Geometry check sheet. Reference: the model listing, model coordinates, mm. Give positions to 0.01 mm unless a question says otherwise; leave off trailing zeros. Order: outer loops, then holes, each group sorted by start corner. A loop starts at its lowest first (then second) coordinate and runs counter-clockwise, first axis right, second up.
```python
from build123d import *

# Parameters (mm, degrees)
F0_R           = 27.4134107223
F1_DEPTH       = 25
F2_R           = 5
F3_DEPTH       = 25
F3_DEPTH_BACK  = 25
F4_R           = 5
F5_R           = 5.7754961782
F6_DEPTH       = 27.4144107223
F6_DEPTH_BACK  = 27.4144107223
F9_R           = 5
F10_DEPTH      = 38.7694173758
F10_DEPTH_BACK = 38.7694173758


with BuildPart() as f1:
    # F0 (on Front) → F1 (new body)
    with BuildSketch(Plane.XZ):
        Circle(F0_R)
    extrude(amount=F1_DEPTH)

    # F2 (on face) → F3 (cut, two sides)
    with BuildSketch(Plane.XZ.offset(25)) as f3_sk:
        with Locations((0, -0.6682850071)):
            Circle(F2_R)
    extrude(amount=-F3_DEPTH, mode=Mode.SUBTRACT)
    extrude(f3_sk.sketch, amount=F3_DEPTH_BACK, mode=Mode.SUBTRACT)

    # F4
    f4_edges = [f1.edges().sort_by_distance(p)[0] for p in [
        (-5, -25, -0.668285),
    ]]
    fillet(f4_edges, radius=F4_R)

    # F5 (on Right) → F6 (cut, two sides)
    with BuildSketch(Plane.YZ) as f6_sk:
        with Locations((-12.5455856323, 0)):
            Circle(F5_R)
    extrude(amount=F6_DEPTH, mode=Mode.SUBTRACT)
    extrude(f6_sk.sketch, amount=-F6_DEPTH_BACK, mode=Mode.SUBTRACT)

    # F9 (on face) → F10 (cut, two sides)
    with BuildSketch(Plane(origin=(0, 0, 0), x_dir=(0, 1, 0), z_dir=(0.7071067812, 0, -0.7071067812))) as f10_sk:
        with Locations((-10, 0)):
            Circle(F9_R)
    extrude(amount=-F10_DEPTH, mode=Mode.SUBTRACT)
    extrude(f10_sk.sketch, amount=F10_DEPTH_BACK, mode=Mode.SUBTRACT)


solid = f1.part
```
Q1. Cross-section at C-C, the plane x = 15. Give the number of separate pieces and of enclosed holes in the cut face, and give its area (3 significant figures).
Q2. Cross-section at A-A, the plane y = -9.25. Record the boundary of the cut face in (x, z).
Q3. Gauge pin test, flat ends, axial feed: P1, Ø6, axis at x = 3, y = -18.5, coming from the +Z side; P2, Ø11.5, axis at x = 0, z = -0.67, coming from the -Y side; P3, Ø1, axis at x = 8.5, y = -9.5, coming from the +Z side; P4, Ø10.5, axis at y = -12.55, z = 0, coming from the +X side. Record the tip position at first contact, or that the pin passes through.
Q4. Release check for a two-part mould opening along X. For faces 1 (the face through (-8.773, -7.312, 14.736)), 2 (the face through (25.323, -12.325, -10.499)), 3 (the face through (0, -25, -12)), 4 (the face through (9.3, -7.69, -15.57)) record: pulls with the +X half, pulls with the -X half, needs draft (parallel to the pull), parting line crosses it, or undercut.
Q5. Thickness scan on L1, parallel to Z at x = 0, y = -18.5; L2, parallel to Y at x = 20, z = 0; L3, parallel to Z at x = -12.5, y = -15.5. Record the ranges inside material, lowest first.
Q6. Cross-section at B-B, the plane y = -3.75. Record the boundary of the cut face in (x, z).
Answers follow:
1. separate pieces: 1
1. enclosed holes: 2
1. area: 931 mm2
2. outline: (-27, -4.74) arc R27.41 ccw to (15.57, -22.56) - (-1.58, -5.41) arc R5 cw to (-2.9, -4.74) - close; (-27, 4.74) - (-11.73, 4.74) - (-22.56, 15.57) arc R27.41 ccw to start; (-15.57, 22.56) - (2.25, 4.74) - (27, 4.74) arc R27.41 ccw to start; (11.73, -4.74) - (22.56, -15.57) arc R27.41 ccw to (27, -4.74) - close
3. P1: stops at z = 27.41
3. P2: stops at y = -22.64
3. P3: stops at z = 26.22
3. P4: passes through
4. face 1: undercut
4. face 2: parting line crosses it
4. face 3: needs draft
4. face 4: undercut
5. L1: z = -27.41 to -5.67, 4.33 to 27.41
5. L2: y = -25 to -18.32, -6.77 to 0
5. L3: z = -24.4 to -4.96, 4.96 to 24.4
6. outline: circle Ø54.83 at (0, 0); hole circle Ø10 at (0, -0.67)
